Geometry: final body of the model. Coordinates: model frame, mm. A direction names the side the tool comes from. Give positions to 0.01 mm unless a question says otherwise; leave off trailing zeros. Write each loop counter-clockwise with the first axis right and the second up, starting at its lowest first coordinate (ties: lowest second). Pieces come first, ordered by that corner, then holes.
```python
from build123d import *

# Parameters (mm, degrees)
HEX1_DEPTH         = 5.461
HEX2_DEPTH         = 8.128
BODYFILLET_R       = 0.889
DSCH_R             = 6.35
CUT_EXTRUDED_DEPTH = 22.86
SKETCH_E_R         = 5.207
CUT_EXTRUDEE_DEPTH = 26.162


with BuildPart() as part:
    # BodySch → Body (revolve)
    with BuildSketch(Plane.XY, mode=Mode.PRIVATE) as body_sk:
        Polygon((-49.022, 0), (-49.022, 11.1125), (-41.3766, 11.1125), (-41.3766, 8.89), (-27.178, 8.89), (-27.178, 10.668), (-19.05, 10.668), (0, 10.074876486), (0, 0), align=None)
    revolve(body_sk.sketch.rotate(Axis((-103.68469285, 0, 0), (1, 0, 0)), 90), axis=Axis((-103.68469285, 0, 0), (1, 0, 0)))

    # Hex1Sch_G → Hex1 (add, symmetric)
    with BuildSketch(Plane(origin=(-41.3766, 0, 0), x_dir=(0, 0, -1), z_dir=(1, 0, 0))):
        Polygon((12.831609733, 0), (6.415804866, 11.1125), (-6.415804866, 11.1125), (-12.831609733, 0), (-6.415804866, -11.1125), (6.415804866, -11.1125), align=None)
    extrude(amount=HEX1_DEPTH, both=True)

    # Hex2Sch_F → Hex2 (add)
    with BuildSketch(Plane.ZY.offset(27.178)):
        Polygon((12.831609733, 0), (6.415804866, 11.1125), (-6.415804866, 11.1125), (-12.831609733, 0), (-6.415804866, -11.1125), (6.415804866, -11.1125), align=None)
    extrude(amount=-HEX2_DEPTH)

    # BodyFillet
    bodyfillet_edges = [part.edges().sort_by_distance(p)[0] for p in [
        (-49.022, 0, -11.1125),
    ]]
    fillet(bodyfillet_edges, radius=BODYFILLET_R)

    # HexfilletSch → Hexfillet (revolve, cut)
    with BuildSketch(Plane(origin=(0, 0, 0), x_dir=(1, 0, 0), z_dir=(0, 1, 0)), mode=Mode.PRIVATE) as hexfillet_sk:
        Polygon((-46.8376, 11.227658516), (-45.911558333, 12.831609733), (-46.8376, 12.831609733), align=None)
        Polygon((-35.9156, 11.227658516), (-36.841641667, 12.831609733), (-35.9156, 12.831609733), align=None)
    revolve(hexfillet_sk.sketch.rotate(Axis((-41.994761709, 0, 0), (1, 0, 0)), 150), axis=Axis((-41.994761709, 0, 0), (1, 0, 0)), mode=Mode.SUBTRACT)

    # DSch → Cut-ExtrudeD (cut)
    with BuildSketch(Plane(origin=(-49.022, 0, 0), x_dir=(0, 0, -1), z_dir=(1, 0, 0))):
        Circle(DSCH_R)
    extrude(amount=CUT_EXTRUDED_DEPTH, mode=Mode.SUBTRACT)

    # Sketch E → Cut-ExtrudeE (cut)
    with BuildSketch(Plane(origin=(0, 0, 0), x_dir=(0, 0, -1), z_dir=(1, 0, 0))):
        Circle(SKETCH_E_R)
    extrude(amount=-CUT_EXTRUDEE_DEPTH, mode=Mode.SUBTRACT)


solid = part.part
```
Item 1: Section C-C, the plane x = -12.5. Return the cut outline in (y, z).
Found:
outline: circle Ø20.93 at (0, 0); hole circle Ø10.41 at (0, 0)
Item 2: Pull-direction query (X, two-part tool) for faces 1 (the face through (-35.916, -9, 1)), 2 (the face through (-46.574, 10.15, 5.788)), 3 (the face through (-23.2, 5.6, -9.6)); classes: +X half, -X half, draft (parallel to the pull), parting line (faces both ways), or undercut.
Found:
face 1: undercut
face 2: -X half
face 3: draft
Item 3: Reachability of faces 4 (the face through (-47.5, -7.5, -8.2)), 5 (the face through (-36.18, -10.15, -5.79)), 6 (the face through (-19.05, 3.3, 10.4)), 7 (the face through (-36.18, 10.15, 5.79)) from +Z, -Z, +X, -X, +Y, -Y: full face, straight path, thin tool, end or side. Return the list, or none.
Found:
face 4: -X
face 5: -Z, -Y
face 6: +X
face 7: +Z, +Y
Item 4: Section B-B, the plane x = -43.5. Return the cut outline in (y, z), plus the area to 3 significant figures.
Found:
outline: (-11.11, -6.42) - (0, -12.83) - (11.11, -6.42) - (11.11, 6.42) - (0, 12.83) - (-11.11, 6.42) - close; hole circle Ø12.7 at (0, 0)
area: 301 mm2
Item 5: Section A-A, the plane x = -25. Return the cut outline in (y, z), plus the area to 3 significant figures.
Found:
outline: (-11.11, -6.42) - (0, -12.83) - (11.11, -6.42) - (11.11, 6.42) - (0, 12.83) - (-11.11, 6.42) - close; hole circle Ø10.41 at (0, 0)
area: 343 mm2
Item 6: Pin query (flat end, axial travel): pin 1 Ø3 at (x, y) = (-15.5, -7) entering from +Z; pin 2 Ø9.5 at (y, z) = (0, 0) entering from +X (1 decimal); pin 3 Ø1.5 at (x, y) = (-6, -1.5) entering from -Z; pin 4 Ø3 at (x, z) = (-37.5, -8) entering from +Y. Return the tip coordinate at first contact, or that it passes through.
Found:
pin 1: stops at z = 9.01
pin 2: passes through
pin 3: stops at z = -10.24
pin 4: stops at y = 10.97
Item 7: Line query: L1, parallel to X at y = 5, z = 7.5; L2, parallel to X at y = 5.25, z = 3.5; L3, parallel to Y at x = -40.5, z = -3. Output: solid intervals per line, ascending.
Found:
L1: x = -49.02 to -35.92, -27.18 to 0
L2: x = -26.16 to 0
L3: y = -11.11 to -5.6, 5.6 to 11.11
